Autodesk Inventor part; units mm, degrees
ref_plane "YZ Plane" through (0, 0, 0) normal (1, 0, 0) x (0, 1, 0)
ref_plane "XZ Plane" through (0, 0, 0) normal (0, 1, 0) x (-1, 0, 0)
ref_plane "XY Plane" through (0, 0, 0) normal (0, 0, 1) x (1, 0, 0)
sketch "Sketch1" plane through (0, 0, 0) normal (0, 1, 0) x (-1, 0, 0)
  line L0 (63.5, 19.05) -> (-63.5, 19.05)
  line L1 (-63.5, 19.05) -> (-63.5, -19.05)
  line L2 (-63.5, -19.05) -> (63.5, -19.05)
  line L3 (63.5, -19.05) -> (63.5, 19.05)
  line L4 (63.5, 19.05) -> (-63.5, -19.05) construction
  line L5 (-63.5, 19.05) -> (63.5, -19.05) construction
  point P0 (0, 0)
  dimension "baseLength" = 127
  dimension "width" = 38.1
extrude "Extrusion1" add sketch "Sketch1" along normal blind 46.0375
sketch "Sketch6" plane through (0, 46.0375, 0) normal (0, 1, 0) x (1, 0, 0)
  line L0 (0, 19.05) -> (-98.425, 19.05)
  line L1 (-98.425, 19.05) -> (-98.425, -19.05)
  line L2 (-98.425, -19.05) -> (-85.725, -19.05)
  line L3 (-85.725, -19.05) -> (-85.725, 6.35)
  line L4 (-85.725, 6.35) -> (0, 6.35)
  line L5 (0, 19.05) -> (0, 6.35) construction
  line L6 (0, 19.05) -> (98.425, 19.05)
  line L7 (98.425, 19.05) -> (98.425, -19.05)
  line L8 (98.425, -19.05) -> (85.725, -19.05)
  line L9 (85.725, -19.05) -> (85.725, 6.35)
  line L10 (85.725, 6.35) -> (0, 6.35)
  line L11 (63.5, 19.05) -> (-63.5, 19.05) construction
  line L12 (-63.5, 19.05) -> (63.5, 19.05) construction
  point P0 (0, 0)
  dimension "d29" = 98.425
  dimension "d30" = 38.1
  dimension "d31" = 12.7
  dimension "interiorWidthForBattery" = 25.4
extrude "Extrusion4" add sketch "Sketch6" along normal blind 25.4
sketch "Sketch7" plane through (-63.5, 0, 19.05) normal (0, 0, 1) x (1, 0, 0)
  line L0 (63.5, 0) -> (63.5, 46.0375) construction
  line L1 (0, 46.0375) -> (127, 46.0375) construction
  line L2 (0, 0) -> (0, 46.0375)
  line L3 (0, 0) -> (19.05, 0)
  line L4 (19.05, 0) -> (19.05, 19.05)
  line L5 (19.05, 19.05) -> (0, 19.05)
  line L6 (0, 19.05) -> (0, 0)
  line L7 (127, 0) -> (107.95, 0)
  line L8 (107.95, 0) -> (107.95, 19.05)
  line L9 (107.95, 19.05) -> (127, 19.05)
  line L10 (127, 19.05) -> (127, 0)
  dimension "d35" = 19.05
  dimension "d47" = 19.05
  dimension "d48" = 19.05
  dimension "d49" = 19.05
extrude "Extrusion5" add sketch "Sketch7" along normal blind 25.4
sketch "Sketch8" plane through (0, 71.4375, 0) normal (0, 1, 0) x (1, 0, 0)
  line L0 (98.425, 19.05) -> (-98.425, 19.05)
  point P0 (0, 0)
  point P1 (0, 12.7)
  dimension "d39" = 6.35
hole "Hole2" at (0, 71.4375, -12.7) direction (0, -1, 0) diameter 10.0838 end through all
sketch "Sketch9" plane through (-63.5, 46.0375, 19.05) normal (0, 0, 1) x (1, 0, 0)
  line L0 (0, 0) -> (127, 0) construction
  line L1 (63.5, -46.0375) -> (38.1, -46.0375)
  line L2 (38.1, -46.0375) -> (38.1, 0)
  line L3 (38.1, 0) -> (63.5, 0)
  line L4 (63.5, -46.0375) -> (63.5, 0) construction
  line L5 (19.05, -46.0375) -> (107.95, -46.0375) construction
  line L6 (127, 0) -> (0, 0) construction
  line L7 (127, 0) -> (0, 0) construction
  line L8 (63.5, -46.0375) -> (88.9, -46.0375)
  line L9 (88.9, -46.0375) -> (88.9, 0)
  line L10 (88.9, 0) -> (63.5, 0)
extrude "Extrusion6" cut sketch "Sketch9" against normal blind 25.4
equation "\"d29\" = batterySupportWall + 0.5 * widthForBattery"
equation "\"d30\" = exteriorWidthForBattery"
equation "\"d31\" = batterySupportWall"
equation "\"widthForBattery\" = 171.45"
equation "\"sideLenghtForBattery\" = 25.4"
equation "\"exteriorWidthForBattery\" = 38.1"
equation "\"batterySupportWall\" = 12.7"
properties part number "BatteryHolder"
Can you work these out from the model? Positions are in its coordinate system, mm. A direction names the side the tool comes from. Round coordinates to 2 decimals unless told otherwise and drop trailing zeros. Loops run counter-clockwise (first coordinate to the right, second up) from the corner with the lowest first, then second, coordinate; pieces in that order, holes last. Notation, with made-up numbers: (48.25, -32) - (87.25, -32) arc R24 ccw to (87.25, -20) - close; hole circle Ø1 at (72, 29). An arc over 180 degrees is marked (long way). Answer in a Markdown table with one row per item. Add a question column.
Q1. I want a section at A-A on z = -12.7. List the corners of the cut face in (x, y) for me (1 decimal), and give its area (3 significant figures).
Q2. I want a section at D-D on z = -2. List the corners of the cut face in (x, y) for me (1 decimal).
Q3. I want a section at B-B on y = 53. List the corners of the cut face in (x, z) for me (3 decimals), and give its area (3 significant figures).
Q4. I need wall thicknesses on L1, parallel to X at y = 20, z = -4; L2, parallel to Z at x = 0, y = 28; L3, parallel to X at y = 14.5, z = -12.7. Which ranges of each line are inside material? Lowest first, please.
Q5. For pin 1 Ø5.5 at (x, z) = (-53.5, 37) entering from +Y; pin 2 Ø11.5 at (x, z) = (0, -12.7) entering from +Y; pin 3 Ø12 at (y, z) = (15, 29) entering from -X; pin 4 Ø14 at (y, z) = (34, 10) entering from +X, each with a flat end and sliding along its axis, tell me the tip position at first contact or that it passes through.
Q6. Which directions (+Z, -Z, +X, -X, +Y, -Y) give clear straight access to the entire face, cutting with the end or side of a thin tool? Please do faces 4 (the flat face through (-44, 46.038, 7)), 5 (the flat face through (25.4, 23, 7)), 6 (the flat face through (54, 19.05, 32)), 7 (the flat face through (-89, 46.038, -5)).
Q7. We'd pull the mould along X, two halves only. Please class faces 1 (the flat face through (92, 59, 19.05)), 2 (the flat face through (63.5, 18, 6)), 3 (the flat face through (-44.45, 9, 32)): pulls with the +X half, pulls with the -X half, needs draft (parallel to the pull), parting line crosses it, or undercut.
Q8. I want a section at C-C on x = 0. List the corners of the cut face in (y, z) for me.
A:
| question | item | result |
|---|---|---|
| 1 | outline | (-98.4, 46) - (-63.5, 46) - (-63.5, 0) - (-5, 0) - (-5, 71.4) - (-98.4, 71.4) - close; (5, 0) - (63.5, 0) - (63.5, 46) - (98.4, 46) - (98.4, 71.4) - (5, 71.4) - close |
| 1 | area | 10,100 mm^2 |
| 2 | outline | (-98.4, 46) - (-85.7, 46) - (-85.7, 71.4) - (-98.4, 71.4) - close; (-63.5, 0) - (-25.4, 0) - (-25.4, 46) - (-63.5, 46) - close; (25.4, 0) - (63.5, 0) - (63.5, 46) - (25.4, 46) - close; (85.7, 46) - (98.4, 46) - (98.4, 71.4) - (85.7, 71.4) - close |
| 3 | outline | (-98.425, -19.05) - (98.425, -19.05) - (98.425, 19.05) - (85.725, 19.05) - (85.725, -6.35) - (-85.725, -6.35) - (-85.725, 19.05) - (-98.425, 19.05) - close; hole circle Ø10.084 at (0, -12.7) |
| 3 | area | 3,070 mm^2 |
| 4 | L1 | -63.5 to -25.4, 25.4 to 63.5 |
| 4 | L2 | -19.05 to -17.74, -7.66 to -6.35 |
| 4 | L3 | -63.5 to -5.04, 5.04 to 63.5 |
| 5 | pin 1 | y = 19.05 |
| 5 | pin 2 | y = 71.44 |
| 5 | pin 3 | x = -63.5 |
| 5 | pin 4 | x = 63.5 |
| 6 | face 4 | +Z, +Y |
| 6 | face 5 | +Z, +Y, -Y |
| 6 | face 6 | +Z, +X, -X, +Y |
| 6 | face 7 | +Z, -Z, -X, -Y |
| 7 | face 1 | needs draft |
| 7 | face 2 | pulls with the +X half |
| 7 | face 3 | undercut |
| 8 | outline | (0, -19.05) - (71.44, -19.05) - (71.44, -17.74) - (0, -17.74) - close; (0, -7.66) - (71.44, -7.66) - (71.44, -6.35) - (0, -6.35) - close |
